Here's how the part is built. I have some questions about the finished solid (model axes, mm). A direction names the side the tool comes from. Round coordinates to 2 decimals unless told otherwise and drop trailing zeros. Order: outer loops, then holes, each group sorted by start corner. A loop starts at its lowest first (then second) coordinate and runs counter-clockwise, first axis right, second up.
```python
from build123d import *

# Parameters (mm, degrees)
SKETCH_1_R      = 29
EXTRUDE_1_DEPTH = 10
SKETCH_2_R      = 18
SKETCH_2_R_2    = 13
EXTRUDE_2_DEPTH = 60
CHAMFER_1_SIZE  = 1


with BuildPart() as part:
    # 草图1 → 凸台-拉伸1 (new body)
    with BuildSketch(Plane(origin=(0, 0, 0), x_dir=(1, 0, 0), z_dir=(0, 1, 0))):
        with Locations(Location((0, 0, 0), (0, 0, 270))):
            Circle(SKETCH_1_R)
    extrude(amount=EXTRUDE_1_DEPTH)

    # 草图2 → 凸台-拉伸2 (add)
    with BuildSketch(Plane(origin=(0, 10, 0), x_dir=(1, 0, 0), z_dir=(0, 1, 0))):
        with Locations(Location((0, 0, 0), (0, 0, 270))):
            Circle(SKETCH_2_R)
        with Locations(Location((0, 0, 0), (0, 0, 270))):
            Circle(SKETCH_2_R_2, mode=Mode.SUBTRACT)
    extrude(amount=EXTRUDE_2_DEPTH)

    # 倒角1
    chamfer_1_edges = [part.edges().sort_by_distance(p)[0] for p in [
        (0, 70, -13),
    ]]
    chamfer(chamfer_1_edges, length=CHAMFER_1_SIZE)


solid = part.part
```
1. If we section it at C-C, the plane z = 0: Write out the boundary of the cut face in (x, y), and give its area (3 significant figures).
Evaluation:
outline: (-29, 0) - (29, 0) - (29, 10) - (18, 10) - (18, 70) - (14, 70) - (13, 69) - (13, 10) - (-13, 10) - (-13, 69) - (-14, 70) - (-18, 70) - (-18, 10) - (-29, 10) - close
area: 1,180 mm2
2. If we section it at D-D, the plane x = 24: Write out the boundary of the cut face in (y, z), and give its area (3 significant figures).
Evaluation:
outline: (0, -16.28) - (10, -16.28) - (10, 16.28) - (0, 16.28) - close
area: 326 mm2
3. If we mould it in two halves opening along X, with no side actions, what happens to faces 3 (the cylindrical face through (-7.91, 39.087, -10.316)), 4 (the cylindrical face through (5.407, 39.58, 17.169)), 5 (the flat face through (0, 0, 0))? For each: released by +X, released by -X, zero draft, split by the parting line, or undercut.
Evaluation:
face 3: undercut
face 4: split by the parting line
face 5: zero draft
4. I need wall thicknesses on probe 1 along X at (y, z) = (31, 0); probe 2 along Y at (x, z) = (22.5, 4.5); probe 3 along X at (y, z) = (63, 4). Which ranges of each line are inside material? Lowest first, please.
Evaluation:
probe 1: x = -18 to -13, 13 to 18
probe 2: y = 0 to 10
probe 3: x = -17.55 to -12.37, 12.37 to 17.55
5. If we section it at A-A, the plane y = 14: Write out the boundary of the cut face in (x, z), and give its area (3 significant figures).
Evaluation:
outline: circle Ø36 at (0, 0); hole circle Ø26 at (0, 0)
area: 487 mm2
6. On a 3-axis mill with a long thin cutter (end or side, diameter ignored), from which of +Z, -Z, +X, -X, +Y, -Y can I reach the whole of each face in a straight line? I mean faces 1 (the flat face through (13.3, 10, 12.5)), 2 (the flat face through (-11, 70, 9)). Say none if no direction works.
Evaluation:
face 1: +Y
face 2: +Z, -Z, +X, -X, +Y
7. I'm going to push flat-ended pins straight in: P1, Ø1.5, axis at y = 26, z = -14, coming from the +X side; P2, Ø5, axis at y = 14, z = -7, coming from the +X side; P3, Ø5, axis at y = 28.5, z = -18.5, coming from the +X side. Where does each tip first touch, or does it pass through?
Evaluation:
P1: stops at x = 12.18
P2: stops at x = 17.43
P3: stops at x = 8.25
8. If we section it at B-B, the plane x = 0: Write out the boundary of the cut face in (y, z), and give its area (3 significant figures).
Evaluation:
outline: (0, -29) - (10, -29) - (10, -18) - (70, -18) - (70, -14) - (69, -13) - (10, -13) - (10, 13) - (69, 13) - (70, 14) - (70, 18) - (10, 18) - (10, 29) - (0, 29) - close
area: 1,180 mm2
